For this review, take the finished solid that the model builds, in its own axes (mm). A direction names the side the tool comes from. Give positions to 0.01 mm unless a question says otherwise; leave off trailing zeros. Loops run counter-clockwise (first coordinate to the right, second up) from the corner with the lowest first, then second, coordinate; pieces in that order, holes last. Notation, with made-up numbers: (39, 50) -> (74, 50) arc R13 cw to (74, 68) -> close; hole circle Ø4 at (-35.75, -0.5). An arc over 180 degrees is marked (long way). Answer as CSV lines item,"result". Start each with the question number.
Item 1: Add section D-D on x = -28.5. State the section outline as (y, z) points (3 decimals).
Item 2: The part is to be moulded in two halves that separate along X. For faces 1 (the face through (14.428, -12, -2)), 2 (the face through (-54.629, 0, 0)), 3 (the face through (86.06, -0.63, -14.26)), say which applies: +X half, -X half, draft (parallel to the pull), parting line (faces both ways), or undercut.
Item 3: Add section B-B on y = -6.25. State how many separate pieces and enclosed holes the cut face has, plus the area to 3 significant figures.
Item 4: Clearance check with flat-ended pins moving along their axes: P1, Ø3, axis at x = 143, z = 8, coming from the -Y side; P2, Ø5, axis at x = 0.5, y = 8, coming from the +Z side; P3, Ø3, axis at x = 170.5, y = -7.5, coming from the +Z side. State where each tip first meets the part, or that it passes through.
Item 5: Add section C-C on x = 173. State the section outline as (y, z) points (3 decimals).
Item 6: Machinability: for faces 4 (the face through (156.92, 7.25, -9.45)), 5 (the face through (-4, 8, -3.175)), 6 (the face through (213, -8, 3.175)), which of the approach directions +Z, -Z, +X, -X, +Y, -Y give a long, thin tool a straight path to every point of the face, cutting with its end or side? Answer none if there is none.
Item 7: Add section A-A on x = 95.5. State the section outline as (y, z) points, plus the area to 3 significant figures.
Item 8: For L1, parallel to Z at x = -32, y = 4.5 (3 decimals); L2, parallel to Y at x = 81.5, z = 8.75; L3, parallel to Z at x = 206, y = 8.25, list the stretches that pass through material, from the lowest coordinate up. Write a range as from..to.
```python
from build123d import *

# Parameters (mm, degrees)
FILLET1_R          = 1.5875
CUT_EXTRUDE1_DEPTH = 3.175
LPATTERN1_COUNT    = 2
LPATTERN1_PITCH    = 31.75
CUT_EXTRUDE2_DEPTH = 3.175


with BuildPart() as part:
    # Sketch1 → Revolve1 (revolve)
    with BuildSketch(Plane.XY, mode=Mode.PRIVATE) as revolve1_sk:
        Polygon((-54.628661224, 0), (-54.628661224, 12.573), (12.046338776, 12.573), (12.046338776, 11.77925), (14.427588776, 11.77925), (14.427588776, 14.2748), (155.715088776, 14.2748), (155.715088776, 11.9126), (158.096338776, 11.9126), (158.096338776, 12.70635), (234.296338776, 12.70635), (234.296338776, 11.2649), (278.746338776, 11.2649), (278.746338776, 0), align=None)
    revolve(revolve1_sk.sketch.rotate(Axis((-43.218877551, 0, 0), (1, 0, 0)), 90), axis=Axis((-43.218877551, 0, 0), (1, 0, 0)))

    # Fillet1
    fillet1_edges = [part.edges().sort_by_distance(p)[0] for p in [
        (-54.628661224, 0, -12.573),
        (278.746338776, 0, -11.2649),
    ]]
    fillet(fillet1_edges, radius=FILLET1_R)

    # Sketch2 → Cut-Extrude1 (cut, symmetric)
    with BuildSketch(Plane.XY):
        with BuildLine():
            Line((-48.022069118, 12.573), (-23.135253331, 12.573))
            ThreePointArc((-23.135253331, 12.573), (-35.578661224, 2.413), (-48.022069118, 12.573))
        make_face()
    cut_extrude1 = extrude(amount=CUT_EXTRUDE1_DEPTH, both=True, mode=Mode.SUBTRACT)

    # LPattern1: Cut-Extrude1 ×2
    with Locations(*[(i * LPATTERN1_PITCH, 0, 0) for i in range(1, LPATTERN1_COUNT)]):
        add(cut_extrude1, mode=Mode.SUBTRACT)

    # Sketch3 → Cut-Extrude2 (cut, symmetric)
    with BuildSketch(Plane.XY):
        with BuildLine():
            Line((162.321680882, -12.70635), (187.208496669, -12.70635))
            ThreePointArc((187.208496669, -12.70635), (174.765088776, -2.54635), (162.321680882, -12.70635))
        make_face()
        with BuildLine():
            Line((200.421680882, -12.70635), (225.308496669, -12.70635))
            ThreePointArc((225.308496669, -12.70635), (212.865088776, -2.54635), (200.421680882, -12.70635))
        make_face()
    extrude(amount=CUT_EXTRUDE2_DEPTH, both=True, mode=Mode.SUBTRACT)


solid = part.part
```
Computed values:
1,outline,"(4.569, -3.175) -> (4.569, 3.175) -> (12.166, 3.175) arc R12.573 ccw (long way) to (12.166, -3.175) -> close"
2,face 1,"undercut"
2,face 2,"-X half"
2,face 3,"draft"
3,separate pieces,"1"
3,enclosed holes,"2"
3,area,"7,470 mm²"
4,P1,"y = -12.71"
4,P2,"z = 11.31"
4,P3,"z = 11.2"
5,outline,"(-12.303, -3.175) arc R12.706 ccw (long way) to (-12.303, 3.175) -> (-2.67, 3.175) -> (-2.67, -3.175) -> close"
6,face 4,"none"
6,face 5,"+Y"
6,face 6,"-Y"
7,outline,"circle Ø28.55 at (0, 0)"
7,area,"640 mm²"
8,L1,"-11.74..-3.175, 3.175..11.74"
8,L2,"-11.28..11.28"
8,L3,"-9.66..9.66"
